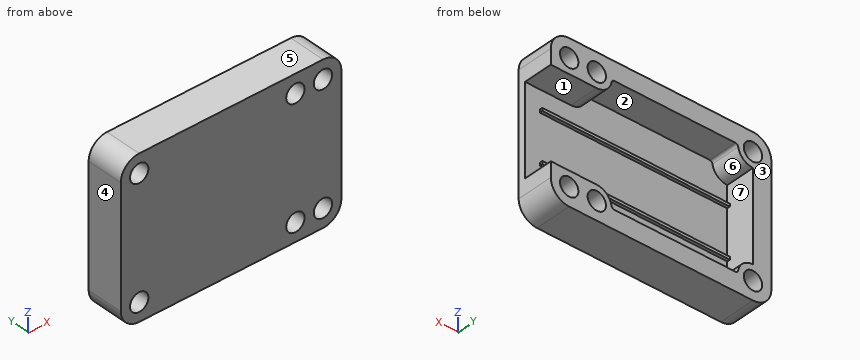
from build123d import *

# Parameters (mm, degrees)
MAIN_BODY_SKETCH_W        = 76.2
MAIN_BODY_SKETCH_H        = 53.975
MAIN_BODY_DEPTH           = 12.7
MOUNTING_HOLES_DEPTH      = 49.386208327
MOUNTING_HOLES_DEPTH_BACK = 49.386208327
MOUNTING_HOLES_SKETCH_R   = 3.175
MAIN_CUTOUT_DEPTH         = 10.16
RIB_SKETCH_W              = 64.77
RIB_SKETCH_H              = 1
RIB_DEPTH                 = 1
OUTER_CORNER_FILLET_R     = 6.35
INNER_CORNER_FILLET_R     = 1


with BuildPart() as part:
    # Main Body Sketch → Main Body (new body)
    with BuildSketch(Plane(origin=(0, 0, 0), x_dir=(1, 0, 0), z_dir=(0, 1, 0))):
        Rectangle(MAIN_BODY_SKETCH_W, MAIN_BODY_SKETCH_H)
    extrude(amount=MAIN_BODY_DEPTH)

    # Mounting Holes Sketch → Mounting Holes (cut, two sides: drawn at the far end of the back side and taken through both)
    with BuildSketch(Plane(origin=(0, 12.7, 0), x_dir=(1, 0, 0), z_dir=(0, 1, 0)).offset(-MOUNTING_HOLES_DEPTH_BACK)):
        with Locations(Location((31.75, -20.6375, 0), (0, 0, 270))):
            Circle(MOUNTING_HOLES_SKETCH_R)
        with Locations(Location((22.225, -20.6375, 0), (0, 0, 270))):
            Circle(MOUNTING_HOLES_SKETCH_R)
        with Locations(Location((-31.75, -20.6375, 0), (0, 0, 270))):
            Circle(MOUNTING_HOLES_SKETCH_R)
        with Locations(Location((31.75, 20.6375, 0), (0, 0, 270))):
            Circle(MOUNTING_HOLES_SKETCH_R)
        with Locations(Location((22.225, 20.6375, 0), (0, 0, 270))):
            Circle(MOUNTING_HOLES_SKETCH_R)
        with Locations(Location((-31.75, 20.6375, 0), (0, 0, 270))):
            Circle(MOUNTING_HOLES_SKETCH_R)
    extrude(amount=MOUNTING_HOLES_DEPTH + MOUNTING_HOLES_DEPTH_BACK, mode=Mode.SUBTRACT)

    # Main Cutout Sketch → Main Cutout (cut)
    with BuildSketch(Plane(origin=(0, 12.7, 0), x_dir=(1, 0, 0), z_dir=(0, 1, 0))):
        with BuildLine():
            Line((31.75, -15.4625), (38.1, -15.4625))
            Line((38.1, -15.4625), (38.1, 15.4625))
            Line((38.1, 15.4625), (22.225, 15.4625))
            ThreePointArc((22.225, 15.4625), (18.565722407, 16.978222407), (17.05, 20.6375))
            Line((17.05, 20.6375), (-26.575, 20.6375))
            ThreePointArc((-26.575, 20.6375), (-28.090722407, 16.978222407), (-31.75, 15.4625))
            Line((-31.75, 15.4625), (-31.75, -15.4625))
            ThreePointArc((-31.75, -15.4625), (-28.090722407, -16.978222407), (-26.575, -20.6375))
            Line((-26.575, -20.6375), (17.05, -20.6375))
            ThreePointArc((17.05, -20.6375), (18.565722407, -16.978222407), (22.225, -15.4625))
            Line((22.225, -15.4625), (31.75, -15.4625))
        make_face()
    extrude(amount=-MAIN_CUTOUT_DEPTH, mode=Mode.SUBTRACT)

    # Rib Sketch → Rib (add)
    with BuildSketch(Plane(origin=(0, 2.54, 0), x_dir=(1, 0, 0), z_dir=(0, 1, 0))):
        with Locations((0.635, -8.5)):
            Rectangle(RIB_SKETCH_W, RIB_SKETCH_H)
        with Locations((0.635, 8.5)):
            Rectangle(RIB_SKETCH_W, RIB_SKETCH_H)
    extrude(amount=RIB_DEPTH)

    # Outer Corner Fillet
    outer_corner_fillet_edges = [part.edges().sort_by_distance(p)[0] for p in [
        (-38.1, 6.35, -26.9875),
        (38.1, 6.35, -26.9875),
        (38.1, 6.35, 26.9875),
        (-38.1, 6.35, 26.9875),
    ]]
    fillet(outer_corner_fillet_edges, radius=OUTER_CORNER_FILLET_R)

    # Inner Corner Fillet
    inner_corner_fillet_edges = [part.edges().sort_by_distance(p)[0] for p in [
        (17.05, 7.62, -20.6375),
        (-26.575, 7.62, -20.6375),
        (-26.575, 7.62, 20.6375),
        (17.05, 7.62, 20.6375),
    ]]
    fillet(inner_corner_fillet_edges, radius=INNER_CORNER_FILLET_R)


solid = part.part
Geometry: final body of the model. Coordinates: model frame, mm. Face numbers are marked on the shaded views. A direction names the side the tool comes from. Round coordinates to 2 decimals unless told otherwise and drop trailing zeros. Loops run counter-clockwise (first coordinate to the right, second up) from the corner with the lowest first, then second, coordinate; pieces in that order, holes last. Notation, with made-up numbers: (-32, -6) -> (-10, -6) arc R26 ccw to (-10, 24) -> close; hole circle Ø5 at (39, -36.5). An arc over 180 degrees is marked (long way). One line per question, with ' | ' between items. Start each with the question number.
1. Section C-C on x = -8. Output: boundary loops of the cut face in (y, z).
2. Mould query, pull axis Z, two halves, no side actions, for the marked faces 4, 5, 6 and 7. Classes: pulls with the +Z half, pulls with the -Z half, needs draft (parallel to the pull), parting line crosses it, or undercut.
3. Line query: line 1 along Z through (x, y) = (-21, 4.25); line 2 along Z through (x, y) = (26, 7.5); line 3 along X through (y, z) = (9.75, -18). Output: solid intervals per line, ascending. Write a range as [from, to].
4. Contact query for flat-ended pins moving along their axis: pin 1 (3 mm diameter, centred on y = 8, z = -1.5, fed in from +X); pin 2 (5 mm diameter, centred on x = 31.75, z = 20.64, fed in from +Y); pin 3 (0.5 mm diameter, centred on y = 3, z = -8.5, fed in from +X); pin 4 (12 mm diameter, centred on x = 4, z = 3.5, fed in from +Y). Output: stop coordinate, or through.
5. Section A-A on x = 23. Output: boundary loops of the cut face in (y, z).
6. Section B-B on y = 7. Count the separate pieces of the cut face and the enclosed holes in it, and give its area (3 significant figures).
7. Section D-D on z = -4.5. Output: boundary loops of the cut face in (x, y), and give its area (3 significant figures).
8. Set-up query: the marked faces 1, 2 and 3. Return all of +Z, -Z, +X, -X, +Y, -Y with unobstructed straight access to the full face (end or side cutting, diameter ignored); none if empty.
Returned:
1) outline: (0, -26.99) -> (12.7, -26.99) -> (12.7, -20.64) -> (2.54, -20.64) -> (2.54, -9) -> (3.54, -9) -> (3.54, -8) -> (2.54, -8) -> (2.54, 8) -> (3.54, 8) -> (3.54, 9) -> (2.54, 9) -> (2.54, 20.64) -> (12.7, 20.64) -> (12.7, 26.99) -> (0, 26.99) -> close
2) face 4: needs draft | face 5: pulls with the +Z half | face 6: undercut | face 7: undercut
3) line 1: z = [-26.99, -20.64], [20.64, 26.99] | line 2: z = [-26.99, -15.46], [15.46, 26.99] | line 3: x = [-38.1, -33.52], [-29.98, -27.3], [17.77, 20.46], [23.99, 29.98], [33.52, 38.1]
4) pin 1: stops at x = -31.75 | pin 2: passes through | pin 3: stops at x = 33.02 | pin 4: stops at y = 3.54
5) outline: (0, -26.99) -> (12.7, -26.99) -> (12.7, -23.72) -> (0, -23.72) -> close; (0, -17.56) -> (12.7, -17.56) -> (12.7, -15.46) -> (2.54, -15.46) -> (2.54, -9) -> (3.54, -9) -> (3.54, -8) -> (2.54, -8) -> (2.54, 8) -> (3.54, 8) -> (3.54, 9) -> (2.54, 9) -> (2.54, 15.46) -> (12.7, 15.46) -> (12.7, 17.56) -> (0, 17.56) -> close; (0, 23.72) -> (12.7, 23.72) -> (12.7, 26.99) -> (0, 26.99) -> close
6) separate pieces: 1 | enclosed holes: 6 | area: 1,250 mm2
7) outline: (-38.1, 0) -> (38.1, 0) -> (38.1, 2.54) -> (-31.75, 2.54) -> (-31.75, 12.7) -> (-38.1, 12.7) -> close | area: 258 mm2
8) face 1: +X, +Y | face 2: +Y | face 3: +Z, -Z, +X, -X, +Y
